Build history of the part. All positions in model axes, mm. A direction names the side the tool comes from. Round coordinates to 2 decimals unless told otherwise and drop trailing zeros. Write each loop counter-clockwise with the first axis right and the second up, starting at its lowest first coordinate (ties: lowest second). Pieces come first, ordered by that corner, then holes. Notation, with made-up numbers: (3.25, 56) -> (24.25, 56) arc R16 cw to (24.25, 81) -> close; hole circle Ø10 at (-13, 36). An arc over 180 degrees is marked (long way). Return JSON: item names as keys, results as strings.
Autodesk Inventor part; units mm, degrees
ref_plane "Work Plane2" through (0, 0, 5.5) normal (0, 0, 1) x (1, 0, 0)
ref_plane "Work Plane8" through (0, 0, 0) normal (0.9396926, 0.3420201, 0) x (0, 0, 1)
ref_plane "Work Plane9" through (0, 0, 0) normal (1, 0, 0) x (0, 1, 0)
sketch "Sketch1" plane through (0, 0, 0) normal (0, 0, 1) x (1, 0, 0)
  circle A0 centre (0, 0) radius 6.4113
  dimension "d0" = 12.8226
extrude "Extrusion1" add sketch "Sketch1" along normal blind 11
ref_plane "Work Plane2" through (0, 0, 5.5) normal (0, 0, 1) x (1, 0, 0)
sketch "Sketch2" plane through (0, 0, 0) normal (0, 0, -1) x (-1, 0, 0)
  circle A0 centre (0, 0) radius 6.4113
  circle A1 centre (0, 0) radius 5.15
  dimension "d3" = 10.3
surface extrude "Pitch Diameter" sketch "Sketch2" against normal through all shown no curves A1
ref_plane "Work Plane8" through (0, 0, 0) normal (0.9396926, 0.3420201, 0) x (0, 0, 1)
ref_plane "Work Plane9" through (0, 0, 0) normal (1, 0, 0) x (0, 1, 0)
spur gear teeth "Spur Gear" teeth 9 pitch diameter 10.125 tip diameter 12.8226 root diameter 7.7817 face width 11 start plane through (0, 0, 0) normal (0, 0, -1) x (-1, 0, 0)
equation "\"d0\" = da_da"
equation "\"d1\" = da_b"
equation "\"d3\" = da_dw"
equation "\"d16\" = da_aw"
equation "\"d43\" = da_aw"
equation "\"d46\" = da_aw"
properties part number "Spur Gear2" material "Steel"
Q1. Two-plate mould, pull along Y, no slides. Class faces 1 (the flat face through (0, 0, 0)), 2 (the cylindrical face through (6.313, 1.121, 5.423)), 3 (the cylindrical face through (-5.55, -3.21, 5.42)), 4 (the cylindrical face through (-5.167, -0.046, 5.423)): +Y half, -Y half, draft (parallel to the pull), parting line (faces both ways), or undercut.
Verdict:
{"face 1": "draft", "face 2": "+Y half", "face 3": "-Y half", "face 4": "undercut"}
Q2. 3-axis set-ups, long thin cutter, end or side, ignore diameter. For faces 5 (the cylindrical face through (-0.01, 6.41, 5.42)), 6 (the flat face through (0, 0, 11)), 7 (the cylindrical face through (0.87, -5.13, 5.42)), 8 (the cylindrical face through (4.84, 1.81, 5.42)), 9 (the cylindrical face through (4.871, -1.724, 5.423)): which of +Z, -Z, +X, -X, +Y, -Y reach the whole face in a straight line?
Verdict:
{"face 5": "+Z, -Z, +Y", "face 6": "+Z, +X, -X, +Y, -Y", "face 7": "+Z, -Z, -Y", "face 8": "+Z, -Z", "face 9": "+Z, -Z, +X"}
Q3. Wall check: L1, parallel to X at y = 5, z = 7.5; L2, parallel to X at y = -3.25, z = 6.5; L3, parallel to Y at x = 3.5, z = 3.75. Give the ranges that are in metal, low to high.
Verdict:
{"L1": "x = -4.01 to -3.23, -0.95 to 0.95, 3.23 to 4.01", "L2": "x = -5.53 to -3.67, -2.26 to 2.26, 3.67 to 5.53", "L3": "y = -3.18 to 1.7, 2.59 to 5.16"}
Q4. Saw through at C-C on y = -4.5. List the corners of the cut face in (x, z), then the cut area to 3 significant figures.
Verdict:
{"outline": "(-2.63, 0) -> (-0.56, 0) -> (-0.56, 11) -> (-2.63, 11) -> close; (0.56, 0) -> (2.63, 0) -> (2.63, 11) -> (0.56, 11) -> close", "area": "45.6 mm²"}
Q5. Saw through at A-A on y = -3. List the corners of the cut face in (x, z).
Verdict:
{"outline": "(-5.67, 0) -> (-3.16, 0) -> (-3.16, 11) -> (-5.67, 11) -> close; (-2.48, 0) -> (2.48, 0) -> (2.48, 11) -> (-2.48, 11) -> close; (3.16, 0) -> (5.67, 0) -> (5.67, 11) -> (3.16, 11) -> close"}
Q6. Pin check, flat tips, straight feed: pin 1 Ø1.5 at (y, z) = (1.5, 7) entering from +X; pin 2 Ø1 at (y, z) = (0, 5.5) entering from -X. Stop position of each tip, or through.
Verdict:
{"pin 1": "stops at x = 6.37", "pin 2": "stops at x = -6.3"}
Q7. Saw through at B-B on x = 5. List the corners of the cut face in (y, z).
Verdict:
{"outline": "(-3.64, 0) -> (-1.83, 0) -> (-1.83, 11) -> (-3.64, 11) -> close; (-0.1, 0) -> (1.81, 0) -> (1.81, 11) -> (-0.1, 11) -> close"}
Q8. Saw through at D-D on y = 4.25. List the corners of the cut face in (x, z).
Verdict:
{"outline": "(-4.44, 0) -> (-2.27, 0) -> (-2.27, 11) -> (-4.44, 11) -> close; (-1.02, 0) -> (1.02, 0) -> (1.02, 11) -> (-1.02, 11) -> close; (2.27, 0) -> (4.44, 0) -> (4.44, 11) -> (2.27, 11) -> close"}
